Source: three-view drawing plus pictorial views. Frame: mm from the lowest corner of the part. Give positions to 0.01 mm unless a question says otherwise; leave off trailing zeros. Order: outer loops, then holes, each group sorted by start corner. A loop starts at its lowest first (then second) coordinate and runs counter-clockwise, first axis right, second up. Notation, with made-up numbers: (55.25, 68) -> (67.25, 68) arc R23 ccw to (67.25, 84) -> close; hole circle Ø3 at (19.25, 89.5). An arc over 180 degrees is marked (long way). Answer in a Markdown table with one row per item. Add a question column.
Q1. Line query: line 1 along Z through (x, y) = (142, 1.3) (1 decimal); line 2 along X through (y, z) = (1.05, 135) (1 decimal); line 3 along X through (y, z) = (0.3, 42) (1 decimal). Output: solid intervals per line, ascending. Write a range as from..to.
Q2. Cut plane C-C on y = 3.7. Count the separate pieces of the cut face and the enclosed holes in it, and give its area (3 significant figures).
Q3. Contact query for flat-ended pins moving along their axis: P1, Ø2, axis at y = 2.5, z = 144.5, coming from the -X side (1 decimal); P2, Ø2.5, axis at x = 131, z = 97.5, coming from the +Y side; P3, Ø3, axis at x = 2.5, y = 3, coming from the -Z side; P4, Ø1, axis at x = 144, y = 3, coming from the -Z side. Output: stop coordinate, or through.
Q4. Cut plane B-B on z = 148. Return the cut outline in (x, y), and give its area (3 significant figures).
Q5. Cut plane A-A on x = 87.5. Return the cut outline in (y, z), and give its area (3 significant figures).
Q6. Cut plane D-D on z = 23. Return the cut outline in (x, y).
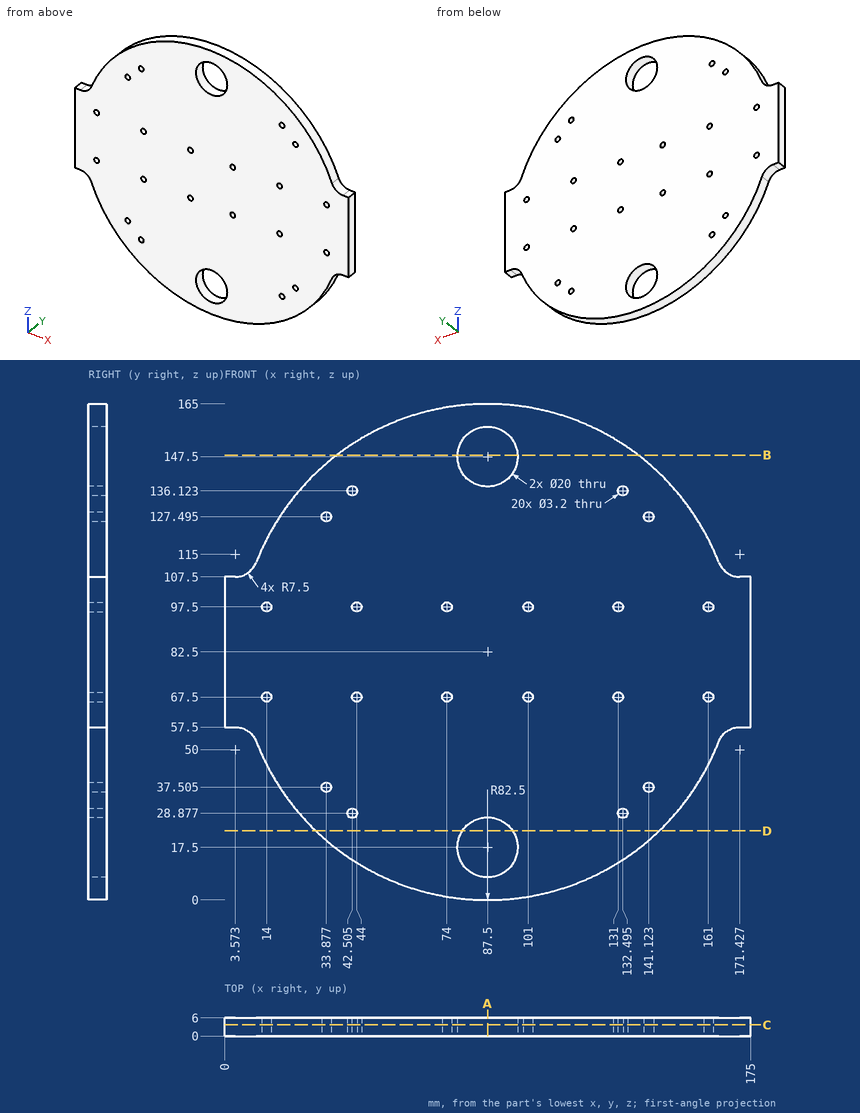
Completed:
| question | item | result |
|---|---|---|
| 1 | line 1 | z = 20.6..36.2, 38.8..126.2, 128.8..144.4 |
| 1 | line 2 | x = 23.9..41.4, 43.6..131.4, 133.6..151.1 |
| 1 | line 3 | x = 15.6..159.4 |
| 2 | separate pieces | 1 |
| 2 | enclosed holes | 22 |
| 2 | area | 21,200 mm² |
| 3 | P1 | stops at x = 32 |
| 3 | P2 | passes through |
| 3 | P3 | stops at z = 57.49 |
| 3 | P4 | stops at z = 21.92 |
| 4 | outline | (37.34, 0) -> (77.51, 0) -> (77.51, 6) -> (37.34, 6) -> close; (97.49, 0) -> (137.66, 0) -> (137.66, 6) -> (97.49, 6) -> close |
| 4 | area | 482 mm² |
| 5 | outline | (0, 0) -> (6, 0) -> (6, 7.5) -> (0, 7.5) -> close; (0, 27.5) -> (6, 27.5) -> (6, 137.5) -> (0, 137.5) -> close; (0, 157.5) -> (6, 157.5) -> (6, 165) -> (0, 165) -> close |
| 5 | area | 750 mm² |
| 6 | outline | (30.35, 0) -> (79.15, 0) -> (79.15, 6) -> (30.35, 6) -> close; (95.85, 0) -> (144.65, 0) -> (144.65, 6) -> (95.85, 6) -> close |
